For this review, take the finished solid that the model builds, in its own axes (mm). A direction names the side the tool comes from. Give positions to 0.01 mm unless a question says otherwise; leave off trailing zeros. Order: outer loops, then holes, each group sorted by start corner. A loop starts at its lowest first (then second) coordinate and runs counter-clockwise, first axis right, second up. Notation, with made-up numbers: (85.5, 26) - (133.5, 26) arc R18 ccw to (133.5, 39) - close; hole circle Ø6 at (80, 86.5). An arc over 180 degrees is marked (long way). One line per item, written item: value.
```python
from build123d import *

# Parameters (mm, degrees)
F0_R     = 6.75
F1_DEPTH = 8
F3_DEPTH = 8.001


with BuildPart() as f1:
    # F0 (on Front) → F1 (new body)
    with BuildSketch(Plane.XZ):
        Circle(F0_R)
    extrude(amount=F1_DEPTH)

    # F2 (on face) → F3 (cut, through all)
    with BuildSketch(Plane.XZ.offset(8)):
        with BuildLine():
            ThreePointArc((-1.4265847744, 0.4635254916), (-1.2924437407, 0.7613075444), (-1.0970305524, 1.0229975401))
            Line((-1.0970305524, 1.0229975401), (-4.0224453589, 3.7509909803))
            ThreePointArc((-4.0224453589, 3.7509909803), (-4.7389603824, 2.7914609963), (-5.2308108396, 1.6995934691))
            Line((-5.2308108396, 1.6995934691), (-1.4265847744, 0.4635254916))
        make_face()
        with BuildLine():
            ThreePointArc((0, 1.5), (0.3246594209, 1.4644440107), (0.6339273926, 1.3594616806))
            Line((0.6339273926, 1.3594616806), (2.3244004396, 4.9846928287))
            ThreePointArc((2.3244004396, 4.9846928287), (1.1904178767, 5.3696280392), (0, 5.5))
            Line((0, 5.5), (0, 1.5))
        make_face()
        with BuildLine():
            ThreePointArc((1.4265847744, 0.4635254916), (1.4815325109, 0.2346516976), (1.5, 0))
            ThreePointArc((1.5, 0), (1.4972021976, -0.0915728093), (1.4888192275, -0.1828040151))
            Line((1.4888192275, -0.1828040151), (5.459003834, -0.6702813887))
            ThreePointArc((5.459003834, -0.6702813887), (5.4897413913, -0.3357669674), (5.5, 0))
            ThreePointArc((5.5, 0), (5.4322858733, 0.8603895577), (5.2308108396, 1.6995934691))
            Line((5.2308108396, 1.6995934691), (1.4265847744, 0.4635254916))
        make_face()
        with BuildLine():
            Line((3.2328188876, -4.4495934691), (0.8816778784, -1.2135254916))
            ThreePointArc((0.8816778784, -1.2135254916), (0.5981236034, -1.3755901116), (0.2862134931, -1.4724407752))
            Line((0.2862134931, -1.4724407752), (1.0494494746, -5.398949509))
            ThreePointArc((1.0494494746, -5.398949509), (2.1931198791, -5.0438304091), (3.2328188876, -4.4495934691))
        make_face()
        with BuildLine():
            Line((-3.2328188876, -4.4495934691), (-0.8816778784, -1.2135254916))
            ThreePointArc((-0.8816778784, -1.2135254916), (-1.1234335812, -0.9939300723), (-1.3119295607, -0.7272144304))
            Line((-1.3119295607, -0.7272144304), (-4.8104083893, -2.6664529114))
            ThreePointArc((-4.8104083893, -2.6664529114), (-4.1192564643, -3.6444102652), (-3.2328188876, -4.4495934691))
        make_face()
    extrude(amount=-F3_DEPTH, mode=Mode.SUBTRACT)


solid = f1.part
```
(1) Take a section at B-B (y = -0.5). Write out the cut boundary in (x, z).
Answers below:
outline: circle Ø13.5 at (0, 0); hole (-5.23, 1.7) - (-1.43, 0.46) arc R1.5 cw to (-1.1, 1.02) - (-4.02, 3.75) arc R5.5 ccw to start; hole (-4.81, -2.67) arc R5.5 ccw to (-3.23, -4.45) - (-0.88, -1.21) arc R1.5 cw to (-1.31, -0.73) - close; hole (0, 1.5) arc R1.5 cw to (0.63, 1.36) - (2.32, 4.98) arc R5.5 ccw to (0, 5.5) - close; hole (0.29, -1.47) - (1.05, -5.4) arc R5.5 ccw to (3.23, -4.45) - (0.88, -1.21) arc R1.5 cw to start; hole (1.43, 0.46) arc R1.5 cw to (1.49, -0.18) - (5.46, -0.67) arc R5.5 ccw to (5.23, 1.7) - close
(2) Machinability: for faces 4 (the face through (0, 0, 0)), 5 (the face through (-3.36, -4.06, 1.09)), which of the approach directions +Z, -Z, +X, -X, +Y, -Y give a long, thin tool a straight path to every point of the face, cutting with its end or side? Answer none if there is none.
Answers below:
face 4: +Z, -Z, +X, -X, +Y
face 5: +Y, -Y
(3) For P1, Ø1, axis at x = -1.5, y = -5, coming from the +Z side; P2, Ø1, axis at x = -3.5, y = -4, coming from the +Z side; P3, Ø4.5, axis at y = -6, z = 4.5, coming from the +X side, all flat-tipped, find the tip position at first contact; note any pin that passes through.
Answers below:
P1: stops at z = 6.68
P2: stops at z = 6.05
P3: stops at x = 6.36
(4) Take a section at A-A (x = -3.75). Write out the cut boundary in (y, z).
Answers below:
outline: (-8, -5.61) - (0, -5.61) - (0, -4.02) - (-8, -4.02) - close; (-8, -2.08) - (0, -2.08) - (0, 1.22) - (-8, 1.22) - close; (-8, 3.5) - (0, 3.5) - (0, 5.61) - (-8, 5.61) - close
(5) Draft analysis for pull direction Z (two halves, no side actions). For faces 1 (the face through (1.47, -4.06, 3.15)), 2 (the face through (-1.46, -3.94, -6.59)), 3 (the face through (0, -8, 0)), state which applies: pulls with the +Z half, pulls with the -Z half, needs draft (parallel to the pull), parting line crosses it, or undercut.
Answers below:
face 1: undercut
face 2: parting line crosses it
face 3: needs draft
(6) Take a section at D-D (x = 3). Write out the cut boundary in (y, z), then the cut area to 3 significant figures.
Answers below:
outline: (-8, -6.05) - (0, -6.05) - (0, -4.61) - (-8, -4.61) - close; (-8, -4.13) - (0, -4.13) - (0, -0.37) - (-8, -0.37) - close; (-8, 0.97) - (0, 0.97) - (0, 6.05) - (-8, 6.05) - close
area: 82.2 mm^2
(7) Wall thickness on line 1 (Z direction, x = -1.25, y = -4.75); line 2 (Z direction, x = -2.75, y = -3); line 3 (X direction, y = -5.5, z = -2.5): over which ranges is each line inside the solid? List them lowest first. Write a range as from..to.
Answers below:
line 1: z = -6.63..-1.72, -0.83..0.83, 1.17..6.63
line 2: z = -6.16..-3.79, -1.52..0.89, 2.56..6.16
line 3: x = -6.27..-4.51, -1.82..0.49, 1.82..6.27
(8) Take a section at C-C (z = 5.75). Write out the cut boundary in (x, y), then the cut area to 3 significant figures.
Answers below:
outline: (-3.54, -8) - (3.54, -8) - (3.54, 0) - (-3.54, 0) - close
area: 56.6 mm^2
